The drawing under review shows one solid part. Ordinate dimensions are in mm from its lowest x, y, z. Coordinates: 2 decimals unless noted, no trailing zeros. Write each loop counter-clockwise with the first axis right and the second up, starting at its lowest first coordinate (ties: lowest second). Pieces come first, ordered by that corner, then holes. Notation, with made-up numbers: (48.25, 40.5) -> (73.25, 40.5) arc R14 ccw to (73.25, 62.5) -> close; hole circle Ø8 at (-24.75, 62.25). An arc over 180 degrees is marked (long way). One line per question, with ' | ' between items. Start each with the question number.
Q1. Add section C-C on z = 1.5. State the section outline as (x, y) points, and give its area (3 significant figures).
Q2. Add section B-B on y = 16. State the section outline as (x, z) points.
Q3. For P1, Ø2.5, axis at x = 31.5, z = 1.5, coming from the +Y side; P2, Ø1.5, axis at y = 51, z = 2, coming from the +X side; P3, Ø0.9, axis at y = 56.5, z = 2, coming from the -X side, all flat-tipped, find the tip position at first contact; note any pin that passes through.
Q4. Wall thickness on probe 1 along X at (y, z) = (36.5, 0.85); probe 2 along Y at (x, z) = (8, 1.25): over which ranges is each line inside the solid? List them lowest first.
Q5. Add section A-A on x = 25.5. State the section outline as (y, z) points.
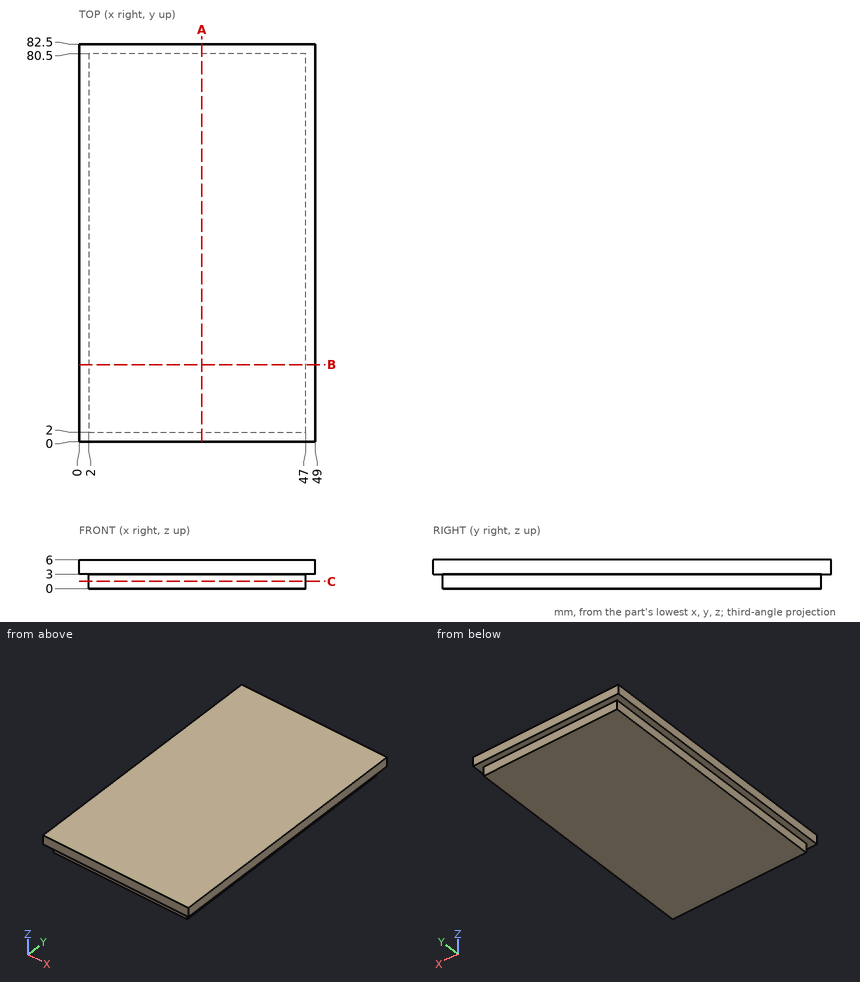
Output values:
1) outline: (2, 2) -> (47, 2) -> (47, 80.5) -> (2, 80.5) -> close | area: 3,530 mm2
2) outline: (0, 3) -> (2, 3) -> (2, 0) -> (47, 0) -> (47, 3) -> (49, 3) -> (49, 6) -> (0, 6) -> close
3) P1: stops at y = 80.5 | P2: stops at x = 47 | P3: stops at x = 2
4) probe 1: x = 2 to 47 | probe 2: y = 2 to 80.5
5) outline: (0, 3) -> (2, 3) -> (2, 0) -> (80.5, 0) -> (80.5, 3) -> (82.5, 3) -> (82.5, 6) -> (0, 6) -> close
